from build123d import *

# Parameters (mm, degrees)
SKETCH1_R           = 5.715
SKETCH1_R_2         = 2.286
BOSS_EXTRUDE1_DEPTH = 7.62
BOSS_EXTRUDE2_START = 12.7
SKETCH2_R           = 2.286
BOSS_EXTRUDE2_DEPTH = 12.7
SKETCH3_R           = 6.35
CUT_EXTRUDE1_DEPTH  = 1.27
SKETCH5_R           = 21.59
CUT_EXTRUDE3_DEPTH  = 7.62
CUT_EXTRUDE2_START  = -15.24
SKETCH4_R           = 4.5466
SKETCH4_R_2         = 4.445
CUT_EXTRUDE2_DEPTH  = 15.24


with BuildPart() as part:
    # Sketch1 → Boss-Extrude1 (new body)
    with BuildSketch(Plane(origin=(0, 0, 0), x_dir=(0, 0, -1), z_dir=(1, 0, 0))):
        with BuildLine():
            Line((2.079548127, 22.50983163), (22.434457752, 15.454797956))
            ThreePointArc((22.434457752, 15.454797956), (27.559, 8.255), (22.434457752, 1.055202044))
            Line((22.434457752, 1.055202044), (2.079548127, -5.99983163))
            ThreePointArc((2.079548127, -5.99983163), (-0.630342168, -6.318636621), (-3.223846154, -5.470769231))
            Line((-3.223846154, -5.470769231), (-19.089076923, 3.878384615))
            ThreePointArc((-19.089076923, 3.878384615), (-21.59, 8.255), (-19.089076923, 12.631615385))
            Line((-19.089076923, 12.631615385), (-3.223846154, 21.980769231))
            ThreePointArc((-3.223846154, 21.980769231), (-0.630342168, 22.828636621), (2.079548127, 22.50983163))
        make_face()
        with Locations(Location((19.939, 8.255, 0), (0, 0, 180))):
            Circle(SKETCH1_R, mode=Mode.SUBTRACT)
        with Locations(Location((0, 16.51, 0), (0, 0, 180))):
            Circle(SKETCH1_R_2, mode=Mode.SUBTRACT)
        with Locations(Location((0, 0, 0), (0, 0, 180))):
            Circle(SKETCH1_R_2, mode=Mode.SUBTRACT)
        with Locations(Location((-16.51, 8.255, 0), (0, 0, 180))):
            Circle(SKETCH1_R_2, mode=Mode.SUBTRACT)
    extrude(amount=BOSS_EXTRUDE1_DEPTH)

    # Sketch2 → Boss-Extrude2 (add)
    with BuildSketch(Plane.ZY.offset(BOSS_EXTRUDE2_START)):
        with BuildLine():
            Line((19.089076923, 12.631615385), (3.223846154, 21.980769231))
            ThreePointArc((3.223846154, 21.980769231), (0.630342168, 22.828636621), (-2.079548127, 22.50983163))
            ThreePointArc((-2.079548127, 22.50983163), (-3.781080863, 21.611561281), (-5.1354637, 20.244904629))
            ThreePointArc((-5.1354637, 20.244904629), (-0.889, 8.255), (-5.1354637, -3.734904629))
            ThreePointArc((-5.1354637, -3.734904629), (-3.781080863, -5.101561281), (-2.079548127, -5.99983163))
            ThreePointArc((-2.079548127, -5.99983163), (0.630342168, -6.318636621), (3.223846154, -5.470769231))
            Line((3.223846154, -5.470769231), (19.089076923, 3.878384615))
            ThreePointArc((19.089076923, 3.878384615), (21.59, 8.255), (19.089076923, 12.631615385))
        make_face()
        Circle(SKETCH2_R, mode=Mode.SUBTRACT)
        with Locations((0, 16.51)):
            Circle(SKETCH2_R, mode=Mode.SUBTRACT)
        with Locations((16.51, 8.255)):
            Circle(SKETCH2_R, mode=Mode.SUBTRACT)
    extrude(amount=-BOSS_EXTRUDE2_DEPTH)

    # Sketch3 → Cut-Extrude1 (cut)
    with BuildSketch(Plane.ZY):
        with Locations((-19.939, 8.255)):
            Circle(SKETCH3_R)
    extrude(amount=-CUT_EXTRUDE1_DEPTH, mode=Mode.SUBTRACT)

    # Sketch5 → Cut-Extrude3 (cut)
    with BuildSketch(Plane.ZY):
        with Locations((-19.939, 8.255)):
            Circle(SKETCH5_R)
    extrude(amount=CUT_EXTRUDE3_DEPTH, mode=Mode.SUBTRACT)

    # Sketch4 → Cut-Extrude2 (cut)
    with BuildSketch(Plane(origin=(7.62, 0, 0), x_dir=(0, 0, -1), z_dir=(1, 0, 0)).offset(CUT_EXTRUDE2_START)):
        Circle(SKETCH4_R)
        with Locations((0, 16.51)):
            Circle(SKETCH4_R_2)
    extrude(amount=CUT_EXTRUDE2_DEPTH, mode=Mode.SUBTRACT)


solid = part.part
Read the model definition and answer for the solid it produces. Units are mm, in the model's axes. A direction names the side the tool comes from. Round coordinates to 2 decimals unless told otherwise and drop trailing zeros. Write each loop counter-clockwise with the first axis right and the second up, starting at its lowest first coordinate (ties: lowest second). Pieces come first, ordered by that corner, then holes. Notation, with made-up numbers: (30.25, -37.5) - (75.25, -37.5) arc R16 ccw to (75.25, -10.5) - close; hole circle Ø3 at (79.25, 71.25). An arc over 180 degrees is marked (long way). One line per question, with ' | ' between items. Start each with the question number.
1. Section A-A (z = 0) is taken. Determine the outline of the cut face in (x, y) (3 decimals), and give its area (3 significant figures).
2. Section B-B (x = -5.25) is taken. Determine the outline of the cut face in (y, z) (3 decimals), and give its area (3 significant figures).
3. Section C-C (y = 9) is taken. Determine the outline of the cut face in (x, z), and give its area (3 significant figures).
4. Each of these flat-tipped pins is pushed along its axis until it touches: pin 1 (6 mm diameter, centred on y = 16.51, z = 0, fed in from +X); pin 2 (10 mm diameter, centred on y = 7.5, z = -18, fed in from -X); pin 3 (1 mm diameter, centred on x = -8.5, y = 17, fed in from -Z). Where does it stop, or does it pass through?
5. For faces 1 (the face through (-3.757, -4.747, -2.703)), 2 (the face through (-10.2, 8.44, -0.89)), 3 (the face through (1.59, 16.71, 4.44)), determine the directions among +Z, -Z, +X, -X, +Y, -Y from which every point of the face is accessible in a straight line to the end or side of a thin tool.
6. For a pull along Y with two mould halves and no side action, classify faces 4 (the face through (-10.2, 2.03, 1.05)), 5 (the face through (3.757, -2.423, -12.399)), 6 (the face through (-12.7, 8, 8)) as +Y half, -Y half, draft (parallel to the pull), parting line (faces both ways), or undercut.
7. Find the intervals of material crossed by probe 1 along Y at (x, z) = (-10.45, 0); probe 2 along Y at (x, z) = (-1, 0) (3 decimals); probe 3 along X at (y, z) = (21, -4), in increasing order. Write a range as [from, to].
8. Section D-D (z = 16.51) is taken. Determine the outline of the cut face in (x, y).
Filled in:
1) outline: (-12.7, -6.35) - (7.62, -6.35) - (7.62, -4.547) - (-7.62, -4.547) - (-7.62, -2.286) - (-12.7, -2.286) - close; (-12.7, 2.286) - (-7.62, 2.286) - (-7.62, 14.224) - (-12.7, 14.224) - close; (-12.7, 18.796) - (-7.62, 18.796) - (-7.62, 20.955) - (7.62, 20.955) - (7.62, 22.86) - (-12.7, 22.86) - close; (0, 4.547) - (7.62, 4.547) - (7.62, 12.065) - (0, 12.065) - close | area: 216 mm²
2) outline: (-5.471, 3.224) arc R6.35 ccw to (-5.451, -3.257) arc R21.59 cw to (-3.999, -2.163) arc R4.547 cw (long way) to (4.358, 1.296) arc R21.59 cw to (12.253, 1.278) arc R4.445 cw (long way) to (20.425, -2.106) arc R21.59 cw to (21.961, -3.257) arc R6.35 ccw to (21.981, 3.224) - (12.632, 19.089) arc R5.08 ccw to (3.878, 19.089) - close; hole circle Ø4.572 at (8.255, 16.51) | area: 314 mm²
3) outline: (-12.7, -0.9) - (-7.62, -0.9) - (-7.62, 1.64) - (0, 1.64) - (0, -13.63) - (1.27, -13.63) - (1.27, -14.27) - (7.62, -14.27) - (7.62, 14.35) - (-12.7, 14.35) - close; (-12.7, 18.67) - (7.62, 18.67) - (7.62, 21.54) - (-12.7, 21.54) - close; (0, -27.52) - (7.62, -27.52) - (7.62, -25.61) - (1.27, -25.61) - (1.27, -26.25) - (0, -26.25) - close | area: 464 mm²
4) pin 1: x = -7.62 | pin 2: x = 0 | pin 3: z = -3.28
5) face 1: -Z | face 2: -Z, -X | face 3: +X
6) face 4: undercut | face 5: -Y half | face 6: draft
7) probe 1: [-6.35, -2.29], [2.29, 14.22], [18.8, 22.86] | probe 2: [-6.35, -4.547], [20.955, 22.86] | probe 3: [-12.7, -7.62], [0, 7.62]
8) outline: (-12.7, 2.36) - (7.62, 2.36) - (7.62, 5.97) - (-12.7, 5.97) - close; (-12.7, 10.54) - (7.62, 10.54) - (7.62, 14.15) - (-12.7, 14.15) - close
